Here's how the part is built. I have some questions about the finished solid (model axes, mm). A direction names the side the tool comes from. Round coordinates to 2 decimals unless told otherwise and drop trailing zeros. Loops run counter-clockwise (first coordinate to the right, second up) from the corner with the lowest first, then second, coordinate; pieces in that order, holes last. Notation, with made-up numbers: M -25.5,20 L -16.5,20 A18 cw -16.5,41 Z; hole C 25.5,-3 d2. An arc over 180 degrees is marked long. Write item = value, one per line. Start each with the question number.
from build123d import *

# Parameters (mm, degrees)
SKETCH_1_R          = 2.9
EXTRUDE_1_DEPTH     = 4
SKETCH_2_W          = 12.628096459
SKETCH_2_H          = 3.5
EXTRUDE_2_DEPTH     = 1
SKETCH_3_R          = 0.5
SKETCH_3_R_2        = 1
CUT_EXTRUDE_1_DEPTH = 5
FILLET_1_R          = 1.5
SKETCH_4_R          = 1.9
CUT_EXTRUDE_2_DEPTH = 3
SKETCH_5_W          = 9.116647883
SKETCH_5_H          = 3.5
CUT_EXTRUDE_3_DEPTH = 2
FILLET_2_R          = 1


with BuildPart() as part:
    # 草图1 → 凸台-拉伸1 (new body)
    with BuildSketch(Plane(origin=(0, 0, 0), x_dir=(1, 0, 0), z_dir=(0, 1, 0))):
        Circle(SKETCH_1_R)
    extrude(amount=EXTRUDE_1_DEPTH)

    # 草图2 → 凸台-拉伸2 (add)
    with BuildSketch(Plane(origin=(0, 0, 0), x_dir=(1, 0, 0), z_dir=(0, 1, 0))):
        with Locations((7.685951771, 0)):
            Rectangle(SKETCH_2_W, SKETCH_2_H)
    extrude(amount=EXTRUDE_2_DEPTH)

    # 草图3 → 切除-拉伸1 (cut, through all)
    with BuildSketch(Plane(origin=(0, 0, 0), x_dir=(1, 0, 0), z_dir=(0, 1, 0))):
        with Locations((8, 0)):
            Circle(SKETCH_3_R)
        with Locations((12, 0)):
            Circle(SKETCH_3_R)
        with Locations((10, 0)):
            Circle(SKETCH_3_R)
        Circle(SKETCH_3_R_2)
        with Locations((4, 0)):
            Circle(SKETCH_3_R)
    extrude(amount=CUT_EXTRUDE_1_DEPTH, mode=Mode.SUBTRACT)

    # 圆角1
    fillet_1_edges = [part.edges().sort_by_distance(p)[0] for p in [
        (14, 0.5, -1.75),
        (14, 0.5, 1.75),
    ]]
    fillet(fillet_1_edges, radius=FILLET_1_R)

    # 草图4 → 切除-拉伸2 (cut)
    with BuildSketch(Plane(origin=(0, 4, 0), x_dir=(1, 0, 0), z_dir=(0, 1, 0))):
        Circle(SKETCH_4_R)
    extrude(amount=-CUT_EXTRUDE_2_DEPTH, mode=Mode.SUBTRACT)

    # 草图5 → 切除-拉伸3 (cut, through all)
    with BuildSketch(Plane(origin=(0, 1, 0), x_dir=(1, 0, 0), z_dir=(0, 1, 0))):
        with Locations((10.558323941, 0)):
            Rectangle(SKETCH_5_W, SKETCH_5_H)
    extrude(amount=-CUT_EXTRUDE_3_DEPTH, mode=Mode.SUBTRACT)

    # 圆角2
    fillet_2_edges = [part.edges().sort_by_distance(p)[0] for p in [
        (6, 0.5, 1.75),
        (6, 0.5, -1.75),
    ]]
    fillet(fillet_2_edges, radius=FILLET_2_R)


solid = part.part
Item 1: I want a section at C-C, the plane y = 0.35. List the corners of the cut face in (x, z) for me.
Item 2: I want a section at D-D, the plane z = 0.9. List the corners of the cut face in (x, y) for me, then the cut area to 3 significant figures.
Item 3: We'd pull the mould along X, two halves only. Please class faces 1 (the cylindrical face through (-1.9, 2.52, -0.08)), 2 (the flat face through (6, 0.5, 0)), 3 (the cylindrical face through (-0.217, 0.493, 0.976)), 4 (the flat face through (1.5, 0, 0)): released by +X, released by -X, zero draft, split by the parting line, or undercut.
Item 4: Please list where these lines run through material, in increasing order: line 1 (X direction, y = 0.35, z = 0); line 2 (Z direction, x = 0, y = 0.25); line 3 (X direction, y = 2.2, z = 0). Write a range as [from, to].
Item 5: I want a section at A-A, the plane z = 0. List the corners of the cut face in (x, y) for me, then the cut area to 3 significant figures.
Item 6: For faces 5 (the flat face through (3.6, 0.5, 1.75)), 6 (the cylindrical face through (3.6, 0.5, 0.3)), 7 (the flat face through (1, 4, 2)), 8 (the flat face through (1, 1, 1)), 9 (the flat face through (3.6, 0.5, -1.75)), which set-ups out of +Z, -Z, +X, -X, +Y, -Y let a thin tool reach every point of the face, with its end or its side?
Item 7: Will these pins go through, and if not, where does the flat tip stop? pin 1 Ø1.8 at (x, z) = (5, 0.5) entering from +Y; pin 2 Ø1.5 at (x, y) = (1.5, 0.5) entering from -Z; pin 3 Ø1.8 at (x, z) = (0, 0) entering from -Y; pin 4 Ø1.1 at (x, y) = (3, 0.5) entering from -Z.
Item 8: I want a section at B-B, the plane x = 4. List the corners of the cut face in (y, z) for me.
Worked out:
q1.outline = M 2.31,-1.75 L 5,-1.75 A1 ccw 6,-0.75 L 6,0.75 A1 ccw 5,1.75 L 2.31,1.75 A2.9 ccw long Z; hole C 0,0 d2; hole C 4,0 d1
q2.outline = M -2.76,0 L -0.44,0 L -0.44,1 L -1.67,1 L -1.67,4 L -2.76,4 Z; M 0.44,0 L 5.99,0 L 5.99,1 L 2.76,1 L 2.76,4 L 1.67,4 L 1.67,1 L 0.44,1 Z
q2.area = 14.4 mm2
q3.face_1 = undercut
q3.face_2 = released by +X
q3.face_3 = undercut
q3.face_4 = zero draft
q4.line_1 = [-2.9, -1], [1, 3.5], [4.5, 6]
q4.line_2 = [-2.9, -1], [1, 2.9]
q4.line_3 = [-2.9, -1.9], [1.9, 2.9]
q5.outline = M -2.9,0 L -1,0 L -1,1 L -1.9,1 L -1.9,4 L -2.9,4 Z; M 1,0 L 3.5,0 L 3.5,1 L 2.9,1 L 2.9,4 L 1.9,4 L 1.9,1 L 1,1 Z; M 4.5,0 L 6,0 L 6,1 L 4.5,1 Z
q5.area = 11.9 mm2
q6.face_5 = +Z, +X, +Y, -Y
q6.face_6 = +Y, -Y
q6.face_7 = +Z, -Z, +X, -X, +Y
q6.face_8 = +Y
q6.face_9 = -Z, +X, +Y, -Y
q7.pin_1 = 1
q7.pin_2 = -2.8
q7.pin_3 = through
q7.pin_4 = -1.75
q8.outline = M 0,-1.75 L 1,-1.75 L 1,-0.5 L 0,-0.5 Z; M 0,0.5 L 1,0.5 L 1,1.75 L 0,1.75 Z
